```python
from build123d import *

# Parameters (mm, degrees)
ESQUISSE1_W             = 268
ESQUISSE1_H             = 70
BOSS_EXTRU_1_DEPTH      = 6
ESQUISSE2_W             = 50
ESQUISSE2_H             = 6
ESQUISSE2_W_2           = 48
ENL_V_MAT_EXTRU_1_DEPTH = 278.055951028
ESQUISSE3_W             = 6
ESQUISSE3_H             = 20
BOSS_EXTRU_2_DEPTH      = 6
ESQUISSE4_R             = 1.5
ESQUISSE4_W             = 40
ESQUISSE4_H             = 15
ENL_V_MAT_EXTRU_2_DEPTH = 10
ESQUISSE5_W             = 6
ESQUISSE5_H             = 19
BOSS_EXTRU_3_DEPTH      = 6
ESQUISSE6_R             = 1.5
ENL_V_MAT_EXTRU_3_DEPTH = 283.863924883
ESQUISSE7_R             = 2.995
ESQUISSE7_R_2           = 3
ENL_V_MAT_EXTRU_4_DEPTH = 3


with BuildPart() as part:
    # Esquisse1 → Boss.-Extru.1 (new body)
    with BuildSketch(Plane.XY):
        with Locations((-134, 35)):
            Rectangle(ESQUISSE1_W, ESQUISSE1_H)
    extrude(amount=BOSS_EXTRU_1_DEPTH)

    # Esquisse2 → Enlèv. mat.-Extru.1 (cut, through all)
    with BuildSketch(Plane.XY.offset(6)):
        with Locations((-243, 3)):
            Rectangle(ESQUISSE2_W, ESQUISSE2_H)
        with Locations((-25, 3)):
            Rectangle(ESQUISSE2_W, ESQUISSE2_H)
        with Locations((-134, 3)):
            Rectangle(ESQUISSE2_W_2, ESQUISSE2_H)
        with Locations((-243, 67)):
            Rectangle(ESQUISSE2_W, ESQUISSE2_H)
        with Locations((-134, 67)):
            Rectangle(ESQUISSE2_W_2, ESQUISSE2_H)
        with Locations((-25, 67)):
            Rectangle(ESQUISSE2_W, ESQUISSE2_H)
    extrude(amount=-ENL_V_MAT_EXTRU_1_DEPTH, mode=Mode.SUBTRACT)

    # Esquisse3 → Boss.-Extru.2 (add)
    with BuildSketch(Plane(origin=(0, 0, 0), x_dir=(0, 0, -1), z_dir=(1, 0, 0))):
        with Locations((-3, 36)):
            Rectangle(ESQUISSE3_W, ESQUISSE3_H)
    extrude(amount=BOSS_EXTRU_2_DEPTH)

    # Esquisse4 → Enlèv. mat.-Extru.2 (cut)
    with BuildSketch(Plane.XY.offset(6)):
        with Locations((-104, 57)):
            Circle(ESQUISSE4_R)
        with Locations((-104, 13)):
            Circle(ESQUISSE4_R)
        with Locations((-10, 57)):
            Circle(ESQUISSE4_R)
        with Locations((-10, 13)):
            Circle(ESQUISSE4_R)
        with Locations((-50, 46.5)):
            Rectangle(ESQUISSE4_W, ESQUISSE4_H)
    extrude(amount=-ENL_V_MAT_EXTRU_2_DEPTH, mode=Mode.SUBTRACT)

    # Esquisse5 → Boss.-Extru.3 (add)
    with BuildSketch(Plane.ZY.offset(268)):
        with Locations((3, 54.5)):
            Rectangle(ESQUISSE5_W, ESQUISSE5_H)
        with Locations((3, 15.5)):
            Rectangle(ESQUISSE5_W, ESQUISSE5_H)
    extrude(amount=BOSS_EXTRU_3_DEPTH)

    # Esquisse6 → Enlèv. mat.-Extru.3 (cut, through all)
    with BuildSketch(Plane(origin=(0, 0, 0), x_dir=(-1, 0, 0), z_dir=(0, 0, -1))):
        with Locations((271, 16)):
            Circle(ESQUISSE6_R)
        with Locations((271, 55)):
            Circle(ESQUISSE6_R)
        with Locations((211, 67)):
            Circle(ESQUISSE6_R)
        with Locations((165, 67)):
            Circle(ESQUISSE6_R)
        with Locations((103, 67)):
            Circle(ESQUISSE6_R)
        with Locations((57, 67)):
            Circle(ESQUISSE6_R)
    extrude(amount=-ENL_V_MAT_EXTRU_3_DEPTH, mode=Mode.SUBTRACT)

    # Esquisse7 → Enlèv. mat.-Extru.4 (cut)
    with BuildSketch(Plane(origin=(0, 0, 0), x_dir=(-1, 0, 0), z_dir=(0, 0, -1))):
        with Locations((271, 16)):
            Circle(ESQUISSE7_R)
        with Locations((271, 55)):
            Circle(ESQUISSE7_R)
        with Locations((211, 67)):
            Circle(ESQUISSE7_R)
        with Locations((165, 67)):
            Circle(ESQUISSE7_R)
        with Locations((103, 67)):
            Circle(ESQUISSE7_R)
        with Locations((57, 67)):
            Circle(ESQUISSE7_R)
        with Locations((104, 57)):
            Circle(ESQUISSE7_R_2)
        with Locations((104, 13)):
            Circle(ESQUISSE7_R_2)
        with Locations((10, 13)):
            Circle(ESQUISSE7_R_2)
        with Locations((10, 57)):
            Circle(ESQUISSE7_R_2)
    extrude(amount=-ENL_V_MAT_EXTRU_4_DEPTH, mode=Mode.SUBTRACT)


solid = part.part
```
Geometry check sheet. Reference: the model listing, model coordinates, mm. A direction names the side the tool comes from. Coordinates: 2 decimals unless noted, no trailing zeros. Loops run counter-clockwise (first coordinate to the right, second up) from the corner with the lowest first, then second, coordinate; pieces in that order, holes last.
Item 1: Access from +Z, -Z, +X, -X, +Y, -Y to the whole of each face (thin tool, end or side, straight path). Record for faces 1 (the face through (-218, 3, 3)), 2 (the face through (3, 26, 3)), 3 (the face through (-10, 60, 1)).
Item 2: Sectioned sample at B-B, the plane z = 1.4. Count the separate pieces of the cut face and the enclosed holes in it, then the cut area to 3 significant figures.
Item 3: Go/stop test with flat-tipped pins: pin 1 Ø3 at (y, z) = (3, 4.5) entering from +X; pin 2 Ø6.5 at (x, y) = (-9, 55.5) entering from -Z; pin 3 Ø1.8 at (x, z) = (-123.5, 2.5) entering from +Y; pin 4 Ø5 at (x, y) = (-271, 16) entering from -Z. Record where each tip stops, or that it passes through.
Item 4: Sectioned sample at A-A, the plane y = 42. Record the boundary of the cut face in (x, z), then the cut area to 3 significant figures.
Item 5: Release check for a two-part mould opening along Y. For faces 4 (the face through (-134, 6, 3)), 5 (the face through (-134, 64, 3)), 6 (the face through (-218, 67, 3)), 7 (the face through (-50, 39, 3)) record: released by +Y, released by -Y, zero draft, split by the parting line, or undercut.
Item 6: Thickness scan on line 1 (X direction, y = 67, z = 5.3); line 2 (Y direction, x = -46, z = 1.6); line 3 (Y direction, x = -61.5, z = 3.7). Record the ranges inside material, lowest first.
Check result:
1. face 1: +Z, -Z, -X, -Y
1. face 2: +Z, -Z, +X, -Y
1. face 3: -Z
2. separate pieces: 1
2. enclosed holes: 11
2. area: 16,400 mm2
3. pin 1: stops at x = -50
3. pin 2: stops at z = 0
3. pin 3: stops at y = 64
3. pin 4: stops at z = 3
4. outline: (-268, 0) - (-70, 0) - (-70, 6) - (-268, 6) - close; (-30, 0) - (6, 0) - (6, 6) - (-30, 6) - close
4. area: 1,400 mm2
5. face 4: released by -Y
5. face 5: released by +Y
5. face 6: zero draft
5. face 7: undercut
6. line 1: x = -218 to -212.5, -209.5 to -166.5, -163.5 to -158, -110 to -104.5, -101.5 to -58.5, -55.5 to -50
6. line 2: y = 6 to 39, 54 to 64
6. line 3: y = 0 to 39, 54 to 70
